Could you check a few things on this drawing? It's one solid part, dimensions in mm from its lowest x, y, z. Coordinates: 2 decimals unless noted, no trailing zeros. Order: outer loops, then holes, each group sorted by start corner. A loop starts at its lowest first (then second) coordinate and runs counter-clockwise, first axis right, second up.
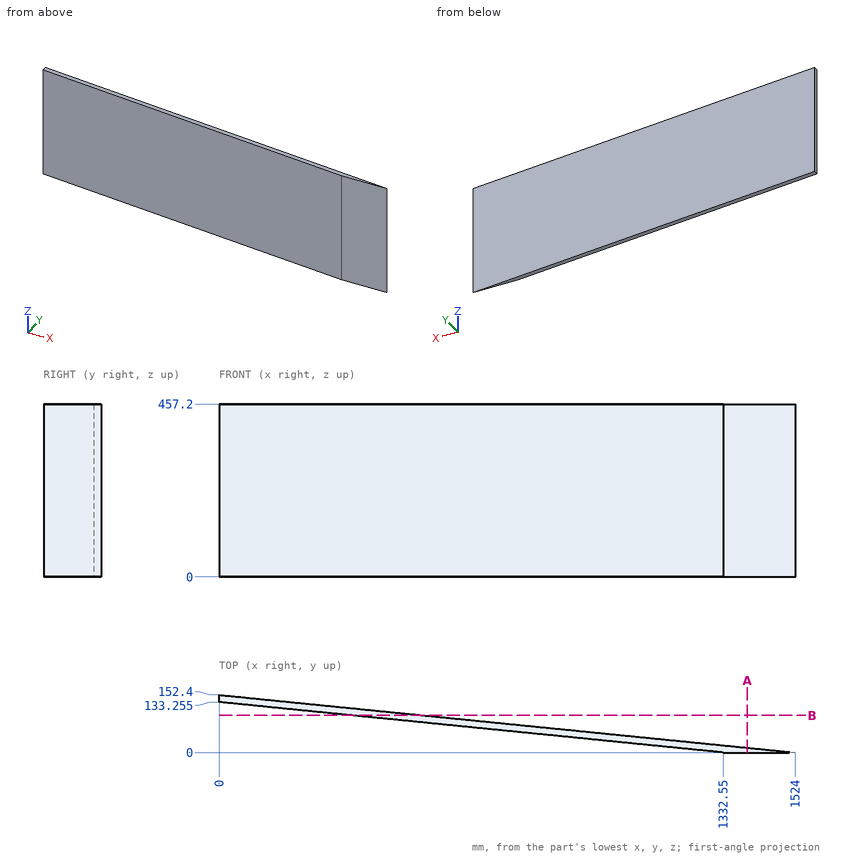
Item 1: Suppose I cut it at A-A (x = 1397). List the corners of the cut face in (y, z) for me.
Item 2: Suppose I cut it at B-B (y = 98). List the corners of the cut face in (x, z) for me.
Item 3: I need wall thicknesses on line 1 (Y direction, x = 212, z = 207.5) (3 decimals); line 2 (Y direction, x = 1430, z = 162). Which ranges of each line are inside material? Lowest first, please.
Item 4: For pin 1 Ø6 at (x, z) = (1176, 200.5) entering from +Y; pin 2 Ø3 at (x, z) = (943.5, 244.5) entering from -Y (3 decimals); pin 3 Ø3 at (x, z) = (975, 81.5) entering from -Y (3 decimals), each with a flat end and sliding along its axis, tell me the tip position at first contact or that it passes through.
Geometry results:
1. outline: (0, 0) - (12.7, 0) - (12.7, 457.2) - (0, 457.2) - close
2. outline: (352.55, 0) - (544, 0) - (544, 457.2) - (352.55, 457.2) - close
3. line 1: y = 112.055 to 131.2
3. line 2: y = 0 to 9.4
4. pin 1: stops at y = 35.1
4. pin 2: stops at y = 38.755
4. pin 3: stops at y = 35.605
